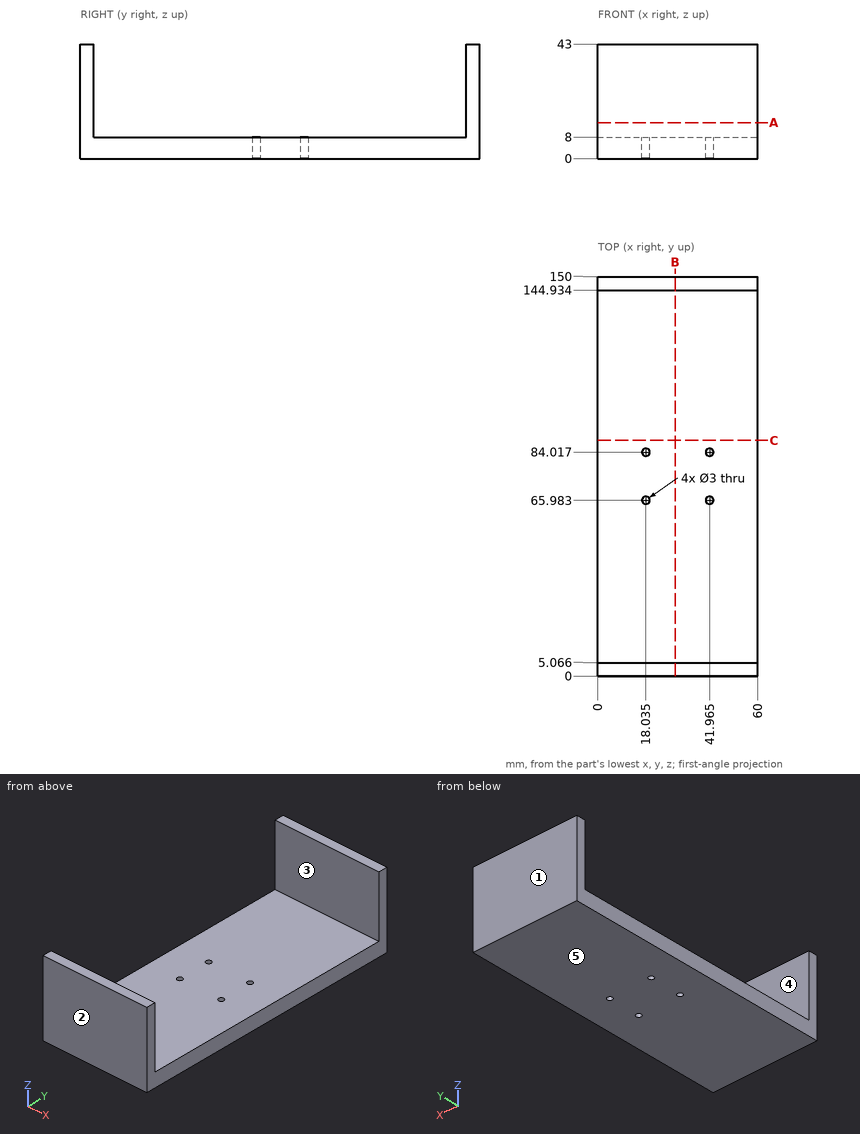
Check sheet for the drawn part. Datum: minimum x, y, z corner. Units: mm. A direction names the side the tool comes from. Round coordinates to 2 decimals unless told otherwise and drop trailing zeros. Order: outer loops, then holes, each group sorted by start corner. A loop starts at its lowest first (then second) coordinate and runs counter-clockwise, first axis right, second up.
1. Section check C-C on y = 88.5. Record the cut outline in (x, z), then the cut area to 3 significant figures.
Final values:
outline: (0, 0) - (60, 0) - (60, 8) - (0, 8) - close
area: 480 mm2
2. Section check A-A on z = 13.5. Record the cut outline in (x, y).
Final values:
outline: (0, 0) - (60, 0) - (60, 5.07) - (0, 5.07) - close; (0, 144.93) - (60, 144.93) - (60, 150) - (0, 150) - close
3. Thickness scan on L1, parallel to Y at x = 57, z = 21; L2, parallel to Z at x = 53, y = 8.5. Record the ranges inside material, lowest first.
Final values:
L1: y = 0 to 5.07, 144.93 to 150
L2: z = 0 to 8
4. Section check B-B on x = 29. Record the cut outline in (y, z).
Final values:
outline: (0, 0) - (150, 0) - (150, 43) - (144.93, 43) - (144.93, 8) - (5.07, 8) - (5.07, 43) - (0, 43) - close
5. Access from +Z, -Z, +X, -X, +Y, -Y to the whole of each face (thin tool, end or side, straight path). Record for the marked faces 4 and 5.
Final values:
face 4: +Z, +X, -X
face 5: -Z, +X, -X, +Y, -Y
6. Release check for a two-part mould opening along Y. For the marked faces 1, 2 and 3 record: +Y half, -Y half, draft (parallel to the pull), parting line (faces both ways), or undercut.
Final values:
face 1: +Y half
face 2: -Y half
face 3: undercut
